```python
from build123d import *

# Parameters (mm, degrees)
CYLINDER002_R     = 19.9
CYLINDER002_DEPTH = 20
FILLET_R          = 2


with BuildPart() as fillet_body:
    # Cylinder002 → Cylinder002 (new body)
    with BuildSketch(Plane.XY.offset(2.5)):
        Circle(CYLINDER002_R)
    extrude(amount=CYLINDER002_DEPTH)

    # Fillet
    fillet_edges = [fillet_body.edges().sort_by_distance(p)[0] for p in [
        (-19.9, 0, 2.5),
    ]]
    fillet(fillet_edges, radius=FILLET_R)


with BuildPart() as fusion:
    # Cone → Cone (revolve)
    with BuildSketch(Plane(origin=(0, 0, 20), x_dir=(1, 0, 0), z_dir=(0, -1, 0))):
        Polygon((0, 0), (7, 0), (10, 10), (0, 10), align=None)
    revolve(axis=Axis((0, 0, 20), (0, 0, 1)))

    # Fusion: union Fillet body
    add(fillet_body.part)


solid = fusion.part
```
Input: part model. Units: mm. Frame: model coordinates. A direction names the side the tool comes from. Coordinates: 2 decimals unless noted, no trailing zeros. Write each loop counter-clockwise with the first axis right and the second up, starting at its lowest first coordinate (ties: lowest second). Pieces come first, ordered by that corner, then holes. Notation, with made-up numbers: (-38.75, -38.75) - (-15.75, -38.75) arc R14 cw to (-15.75, -16.75) - close; hole circle Ø2 at (-25, -19). An arc over 180 degrees is marked (long way). Put each result on its own line as item: value. Start each with the question number.
1) Contact query for flat-ended pins moving along their axis: pin 1 (2 mm diameter, centred on x = -1, z = 16, fed in from -Y); pin 2 (8 mm diameter, centred on x = -15, z = 16.5, fed in from -Y); pin 3 (3 mm diameter, centred on y = 15.5, z = 18, fed in from +X). Output: stop coordinate, or through.
2) Cut plane C-C (z = 7.25). Return the cut outline in (x, y).
3) Reachability of faces 1 (the face through (9, 0, 22.5)), 2 (the face through (-15.8, -12.1, 13.4)) from +Z, -Z, +X, -X, +Y, -Y: full face, straight path, thin tool, end or side. Return the list, or none.
4) Ray query, L1, parallel to Z at x = -15, y = -4; L2, parallel to Y at x = 0, z = 15.25; L3, parallel to Y at x = 3, z = 25.75. Return the intervals inside material, ascending.
5) Cut plane D-D (z = 25). Return the cut outline in (x, y), plus the area to 3 significant figures.
6) Mould query, pull axis Z, two halves, no side actions, for faces 3 (the face through (-1.765, -7.947, 23.803)), 4 (the face through (0, 0, 2.5)), 5 (the face through (0, 0, 30)). Classes: pulls with the +Z half, pulls with the -Z half, needs draft (parallel to the pull), parting line crosses it, or undercut.
7) Cut plane A-A (x = 0). Return the cut outline in (y, z).
Resolved:
1. pin 1: stops at y = -19.9
1. pin 2: stops at y = -16.58
1. pin 3: stops at x = 14.14
2. outline: circle Ø39.8 at (0, 0)
3. face 1: none
3. face 2: +Z, -Z
4. L1: z = 2.5 to 22.5
4. L2: y = -19.9 to 19.9
4. L3: y = -8.19 to 8.19
5. outline: circle Ø17 at (0, 0)
5. area: 227 mm2
6. face 3: undercut
6. face 4: pulls with the -Z half
6. face 5: pulls with the +Z half
7. outline: (-19.9, 4.5) arc R2 ccw to (-17.9, 2.5) - (17.9, 2.5) arc R2 ccw to (19.9, 4.5) - (19.9, 22.5) - (7.75, 22.5) - (10, 30) - (-10, 30) - (-7.75, 22.5) - (-19.9, 22.5) - close
